Design review of the part shown in the three views and the two pictorial views. Dimensions are in mm from the part's minimum x, y and z. A direction names the side the tool comes from. Coordinates: 2 decimals unless noted, no trailing zeros. Loops run counter-clockwise (first coordinate to the right, second up) from the corner with the lowest first, then second, coordinate; pieces in that order, holes last.
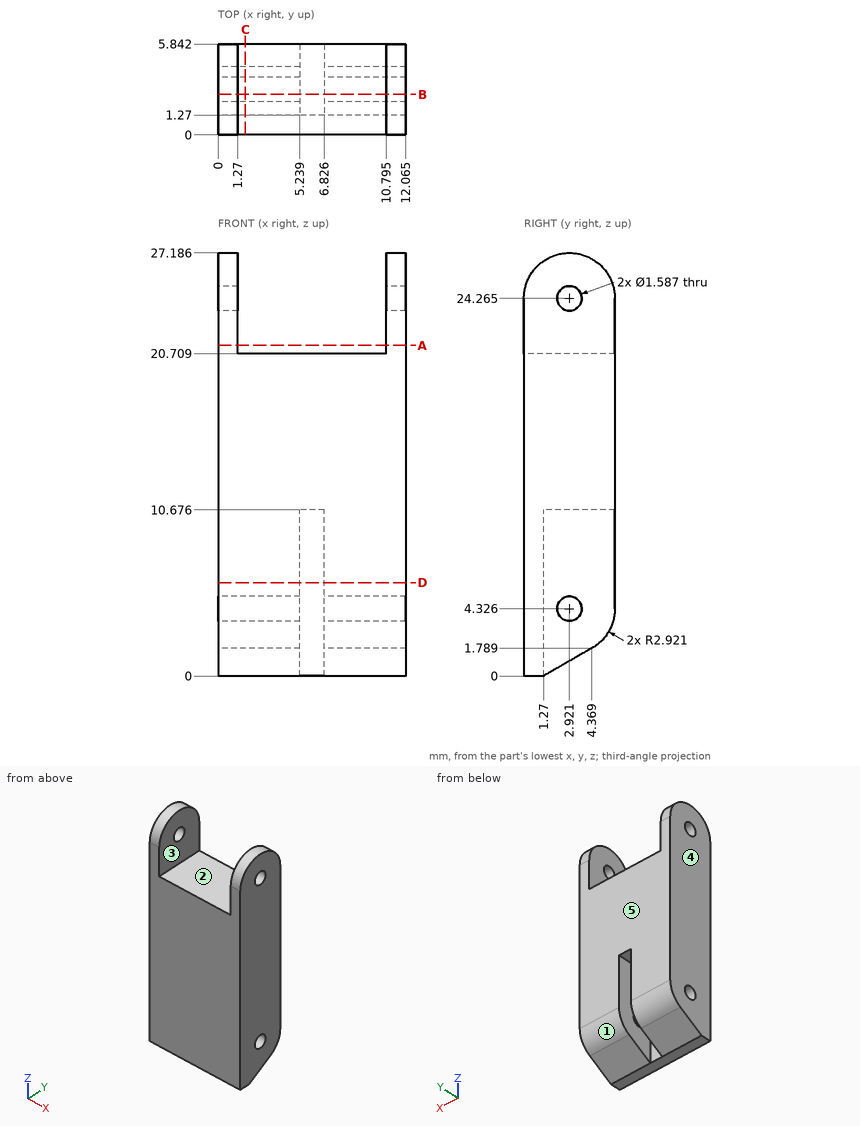
Q1. Consider section C-C (x = 1.75). State the section outline as (y, z) points (1 decimal).
Q2. Consider section D-D (z = 6). State the section outline as (x, y) points (1 decimal).
Q3. The part is to be moulded in two halves that separate along X. For the marked faces 3, 4 and 5, say which applies: +X half, -X half, draft (parallel to the pull), parting line (faces both ways), or undercut.
Q4. Machinability: for the marked faces 1 and 2, which of the approach directions +Z, -Z, +X, -X, +Y, -Y give a long, thin tool a straight path to every point of the face, cutting with its end or side? Answer none if there is none.
Q5. For pin 1 Ø1.4 at (y, z) = (2.92, 24.27) entering from +X; pin 2 Ø3.5 at (y, z) = (2.5, 5.5) entering from -X; pin 3 Ø2 at (x, y) = (7, 3.5) entering from +Z; pin 4 Ø0.8 at (x, z) = (6, 7.5) entering from +Y, all flat-tipped, find the tip position at first contact; note any pin that passes through.
Q6. Wall thickness on probe 1 along X at (y, z) = (4.65, 22.75) (1 decimal); probe 2 along X at (y, z) = (4.3, 10) (1 decimal); probe 3 along Y at (x, z) = (11, 4.5) (1 decimal): over which ranges is each line inside the solid? List them lowest first.
Q7. Consider section B-B (y = 2.6). State the section outline as (x, z) points (1 decimal).
Q8. Consider section A-A (z = 21.25). State the section outline as (x, y) points (1 decimal).
Model answer:
1. outline: (0, 0) - (1.3, 0) - (4.4, 1.8) arc R2.9 ccw to (5.8, 4.3) - (5.8, 20.7) - (0, 20.7) - close; hole circle Ø1.6 at (2.9, 4.3)
2. outline: (0, 0) - (12.1, 0) - (12.1, 5.8) - (6.8, 5.8) - (6.8, 1.3) - (5.2, 1.3) - (5.2, 5.8) - (0, 5.8) - close
3. face 3: undercut
3. face 4: -X half
3. face 5: draft
4. face 1: -Z, +X, -X, +Y
4. face 2: +Z, +Y, -Y
5. pin 1: passes through
5. pin 2: stops at x = 0
5. pin 3: stops at z = 20.71
5. pin 4: stops at y = 1.27
6. probe 1: x = 0 to 1.3, 10.8 to 12.1
6. probe 2: x = 0 to 5.2, 6.8 to 12.1
6. probe 3: y = 0 to 2.1, 3.7 to 5.8
7. outline: (0, 0.8) - (5.2, 0.8) - (5.2, 3.6) - (0, 3.6) - close; (0, 5.1) - (5.2, 5.1) - (5.2, 10.7) - (6.8, 10.7) - (6.8, 5.1) - (12.1, 5.1) - (12.1, 23.5) - (10.8, 23.5) - (10.8, 20.7) - (1.3, 20.7) - (1.3, 23.5) - (0, 23.5) - close; (0, 25) - (1.3, 25) - (1.3, 27.2) - (0, 27.2) - close; (6.8, 0.8) - (12.1, 0.8) - (12.1, 3.6) - (6.8, 3.6) - close; (10.8, 25) - (12.1, 25) - (12.1, 27.2) - (10.8, 27.2) - close
8. outline: (0, 0) - (1.3, 0) - (1.3, 5.8) - (0, 5.8) - close; (10.8, 0) - (12.1, 0) - (12.1, 5.8) - (10.8, 5.8) - close
